Autodesk Inventor part; units mm, degrees
ref_plane "YZ Plane" through (0, 0, 0) normal (1, 0, 0) x (0, 1, 0)
ref_plane "XZ Plane" through (0, 0, 0) normal (0, 1, 0) x (-1, 0, 0)
ref_plane "XY Plane" through (0, 0, 0) normal (0, 0, 1) x (1, 0, 0)
sketch "スケッチ1" plane through (0, 0, 0) normal (0, 0, 1) x (1, 0, 0)
  line L0 (0, 0) -> (25, 0)
  line L1 (25, 0) -> (25, 5)
  line L2 (25, 5) -> (0, 5)
  line L3 (0, 5) -> (0, 0)
  circle A0 centre (5, 2.5) radius 1.5 construction
  circle A1 centre (20, 2.5) radius 1.5 construction
  line L4 (20, 2.5) -> (5, 2.5) construction
  line L5 (-10.9711, 1.5408) -> (-31.4499, -12.7986)
  line L6 (-31.4499, -12.7986) -> (-28.582, -16.8943)
  line L7 (-28.582, -16.8943) -> (-8.1032, -2.5549)
  line L8 (-8.1032, -2.5549) -> (-10.9711, 1.5408)
  line L9 (-30.016, -14.8465) -> (-9.5372, -0.5071) construction
  arc A2 (0, 2.5) -> (-9.5372, -0.5071) centre (0, -14.1275) ccw construction
  arc A3 (0, 5) -> (-10.9711, 1.5408) centre (0, -14.1275) ccw
  arc A4 (0, 0) -> (-8.1032, -2.5549) centre (0, -14.1275) ccw
  circle A5 centre (-25.9202, -11.9786) radius 1.5 construction
  circle A6 centre (-13.6329, -3.3749) radius 1.5 construction
  point P0 (25, 2.5)
  point P1 (-8.1032, -2.5549)
  point P2 (-10.9711, 1.5408)
  dimension "d0" = 5
  dimension "d1" = 3
  dimension "d2" = 3
  dimension "d3" = 15
  dimension "d4" = 5
  dimension "d5" = 5
  dimension "d6" = 5
  dimension "d7" = 25
  dimension "d8" = 2.5
  dimension "d9" = 2.5
  dimension "d10" = 145
  dimension "d11" = 10
  dimension "d12" = 3
  dimension "d13" = 3
  dimension "d14" = 5
  dimension "d15" = 5
extrude "押し出し1" add sketch "スケッチ1" along normal blind 10
sketch "スケッチ2" plane through (0, 0, 0) normal (0, -1, 0) x (1, 0, 0)
  line L0 (25, 0) -> (25, 10)
  circle A0 centre (5, 5) radius 1.5
  circle A1 centre (20, 5) radius 1.5
  point P0 (0, 0)
  point P1 (25, 5)
  dimension "d18" = 3
  dimension "d19" = 3
  dimension "d20" = 15
  dimension "d21" = 5
extrude "押し出し2" cut sketch "スケッチ2" against normal through all
sketch "スケッチ3" plane through (-8.1032, -2.5549, 0) normal (0.5736, -0.8192, 0) x (0.8192, 0.5736, 0)
  line L0 (-25, 0) -> (-25, 10)
  circle A0 centre (-20, 5) radius 1.5
  circle A1 centre (-5, 5) radius 1.5
  point P0 (8.1032, 0)
  point P1 (-25, 5)
  dimension "d24" = 3
  dimension "d25" = 3
  dimension "d26" = 15
  dimension "d27" = 5
extrude "押し出し3" cut sketch "スケッチ3" against normal through all
properties part number "カウンター1.2.1" material "アルミニウム 6061"
Geometry check sheet. Reference: the model listing, model coordinates, mm. A direction names the side the tool comes from. Round coordinates to 2 decimals unless told otherwise and drop trailing zeros. Loops run counter-clockwise (first coordinate to the right, second up) from the corner with the lowest first, then second, coordinate; pieces in that order, holes last. Notation, with made-up numbers: (-30.75, -10.5) - (-19.75, -10.5) arc R11 cw to (-19.75, 3.5) - close; hole circle Ø2 at (9, 63.5). An arc over 180 degrees is marked (long way). Answer as CSV lines item,"result".
(1) Cross-section at A-A, the plane x = 20. Enter the section's corners in (y, z), and give its area (3 significant figures).
Output values:
outline,"(0, 0) - (5, 0) - (5, 3.5) - (0, 3.5) - close; (0, 6.5) - (5, 6.5) - (5, 10) - (0, 10) - close"
area,"35.0 mm²"
(2) Material ranges on line 1 along Z through (x, y) = (-25.5, -12.25); line 2 along Y through (x, z) = (13.5, 9); line 3 along X through (y, z) = (-7.5, 8.5), recorded low to high.
Output values:
line 1,"z = 0 to 3.51, 6.49 to 10"
line 2,"y = 0 to 5"
line 3,"x = -23.88 to -15.17"
(3) Release check for a two-part mould opening along Z. For faces 1 (the face through (6.386, 2.465, 4.425)), 2 (the face through (-14.84, -4.26, 5.07)), 3 (the face through (25, 2, 5)), 4 (the face through (-5, 0, 0)) record: released by +Z, released by -Z, zero draft, split by the parting line, or undercut.
Output values:
face 1,"undercut"
face 2,"undercut"
face 3,"zero draft"
face 4,"released by -Z"
(4) Depth check by flat-ended pin: pin 1 Ø4 at (x, z) = (1.5, 2) entering from -Y; pin 2 Ø1 at (y, z) = (2.5, 7) entering from -X; pin 3 Ø5 at (y, z) = (-9, 2.5) entering from +X. Enter the tip coordinate at first touch or a pass-through.
Output values:
pin 1,"stops at y = -0.01"
pin 2,"stops at x = -10.28"
pin 3,"stops at x = -13.74"
(5) Cross-section at C-C, the plane x = -3. Enter the section's corners in (y, z).
Output values:
outline,"(-0.32, 0) - (4.76, 0) - (4.76, 10) - (-0.32, 10) - close"
(6) Set-up check for faces 5 (the face through (12, 0, 5)), 6 (the face through (-30.036, -14.818, 4.93)): record each of +Z, -Z, +X, -X, +Y, -Y from which the full face is reachable in a straight line by a thin tool's end or side.
Output values:
face 5,"+Z, -Z, +X, -Y"
face 6,"+Z, -Z, -X, -Y"
(7) Cross-section at B-B, the plane z = 5. Enter the section's corners in (x, y), and give its area (3 significant figures).
Output values:
outline,"(-31.45, -12.8) - (-28.58, -16.89) - (-25.71, -14.89) - (-28.58, -10.79) - close; (-26.13, -9.07) - (-23.26, -13.17) - (-13.43, -6.28) - (-16.3, -2.19) - close; (-13.84, -0.47) - (-10.97, -4.56) - (-8.1, -2.55) arc R14.13 cw to (0, 0) - (3.5, 0) - (3.5, 5) - (0, 5) arc R19.13 ccw to (-10.97, 1.54) - close; (6.5, 0) - (18.5, 0) - (18.5, 5) - (6.5, 5) - close; (21.5, 0) - (25, 0) - (25, 5) - (21.5, 5) - close"
area,"241 mm²"
